For this review, use the dimensioned drawing (mm, ordinates from the lowest corner) and the shaded views. A direction names the side the tool comes from. Round coordinates to 2 decimals unless told otherwise and drop trailing zeros. Write each loop counter-clockwise with the first axis right and the second up, starting at its lowest first coordinate (ties: lowest second). Pieces come first, ordered by that corner, then holes.
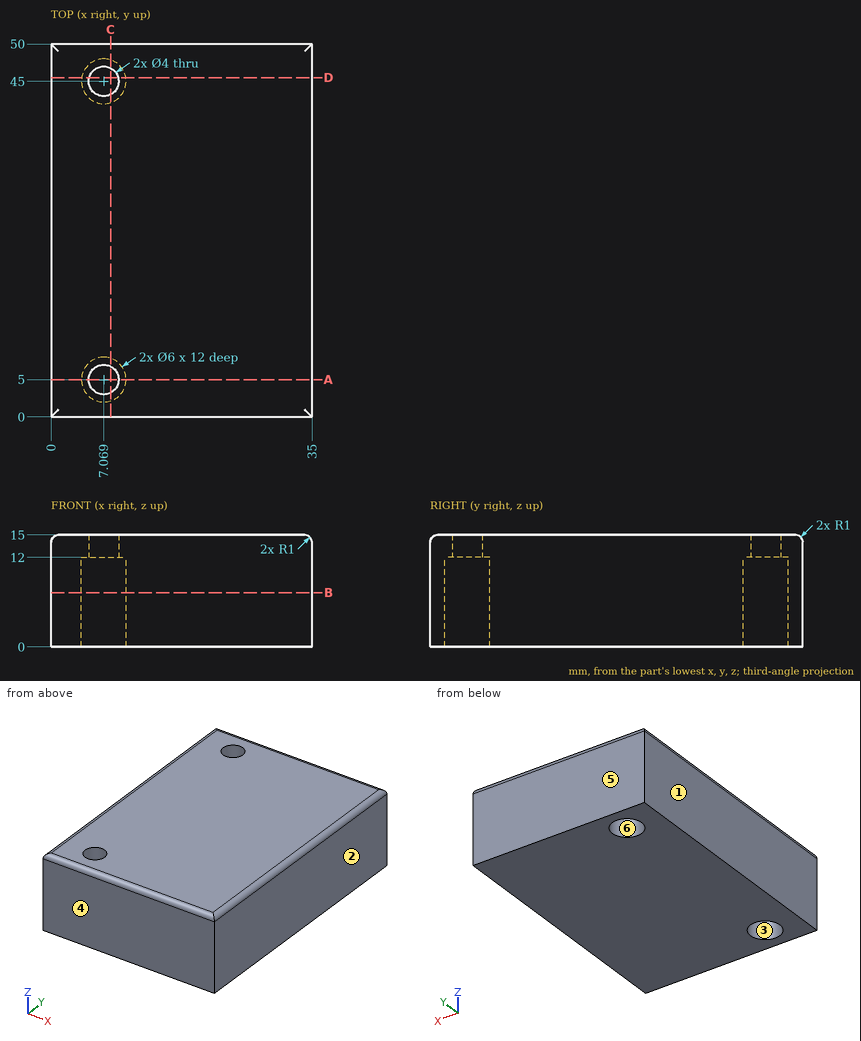
(1) For line 1 along X through (y, z) = (5, 4.5); line 2 along X through (y, z) = (5, 14); line 3 along Y through (x, z) = (5, 9.25), list the stretches that pass through material, from the lowest coordinate up.
Geometry check:
line 1: x = 0 to 4.07, 10.07 to 35
line 2: x = 0 to 5.07, 9.07 to 35
line 3: y = 0 to 2.83, 7.17 to 42.83, 47.17 to 50
(2) We need section A-A, the plane y = 5. Give the boundary of the cut face in (x, z).
Geometry check:
outline: (0, 0) - (4.07, 0) - (4.07, 12) - (5.07, 12) - (5.07, 15) - (1, 15) arc R1 ccw to (0, 14) - close; (9.07, 12) - (10.07, 12) - (10.07, 0) - (35, 0) - (35, 14) arc R1 ccw to (34, 15) - (9.07, 15) - close
(3) For the marked faces 5 and 6, list the 3-axis set-ups (+Z, -Z, +X, -X, +Y, -Y) from which the entire face can be reached by the end or side of a thin tool; tool diameter is ignored.
Geometry check:
face 5: +Z, -Z, +X, -X, +Y
face 6: -Z
(4) For pin 1 Ø6.5 at (x, y) = (7.07, 5) entering from +Z; pin 2 Ø3 at (x, y) = (8, 45) entering from -Z, all flat-tipped, find the tip position at first contact; note any pin that passes through.
Geometry check:
pin 1: stops at z = 15
pin 2: stops at z = 12
(5) Mouldability with a two-part tool opening along X and no side actions: class the marked faces 1, 2, 3 and 4 as pulls with the +X half, pulls with the -X half, needs draft (parallel to the pull), parting line crosses it, or undercut.
Geometry check:
face 1: pulls with the -X half
face 2: pulls with the +X half
face 3: undercut
face 4: needs draft
(6) We need section D-D, the plane y = 45.5. Give the boundary of the cut face in (x, z) (1 decimal), and give its area (3 significant figures).
Geometry check:
outline: (0, 0) - (4.1, 0) - (4.1, 12) - (5.1, 12) - (5.1, 15) - (1, 15) arc R1 ccw to (0, 14) - close; (9, 12) - (10, 12) - (10, 0) - (35, 0) - (35, 14) arc R1 ccw to (34, 15) - (9, 15) - close
area: 442 mm2
(7) We need section B-B, the plane z = 7.25. Give the boundary of the cut face in (x, y), and give its area (3 significant figures).
Geometry check:
outline: (0, 0) - (35, 0) - (35, 50) - (0, 50) - close; hole circle Ø6 at (7.07, 5); hole circle Ø6 at (7.07, 45)
area: 1,690 mm2
(8) We need section C-C, the plane x = 8. Give the boundary of the cut face in (y, z).
Geometry check:
outline: (0, 0) - (2.15, 0) - (2.15, 12) - (3.23, 12) - (3.23, 15) - (1, 15) arc R1 ccw to (0, 14) - close; (6.77, 12) - (7.85, 12) - (7.85, 0) - (42.15, 0) - (42.15, 12) - (43.23, 12) - (43.23, 15) - (6.77, 15) - close; (46.77, 12) - (47.85, 12) - (47.85, 0) - (50, 0) - (50, 14) arc R1 ccw to (49, 15) - (46.77, 15) - close
